Check sheet for the drawn part. Datum: minimum x, y, z corner. Units: mm. A direction names the side the tool comes from. Round coordinates to 2 decimals unless told otherwise and drop trailing zeros. Order: outer loops, then holes, each group sorted by start corner. A loop starts at its lowest first (then second) coordinate and runs counter-clockwise, first axis right, second up. Notation, with made-up numbers: (-21.75, 71.25) -> (22.25, 71.25) arc R31 ccw to (22.25, 98.25) -> close; hole circle Ø1 at (0.5, -25.75). An arc over 180 degrees is marked (long way). Answer in a Markdown table with one row per item.
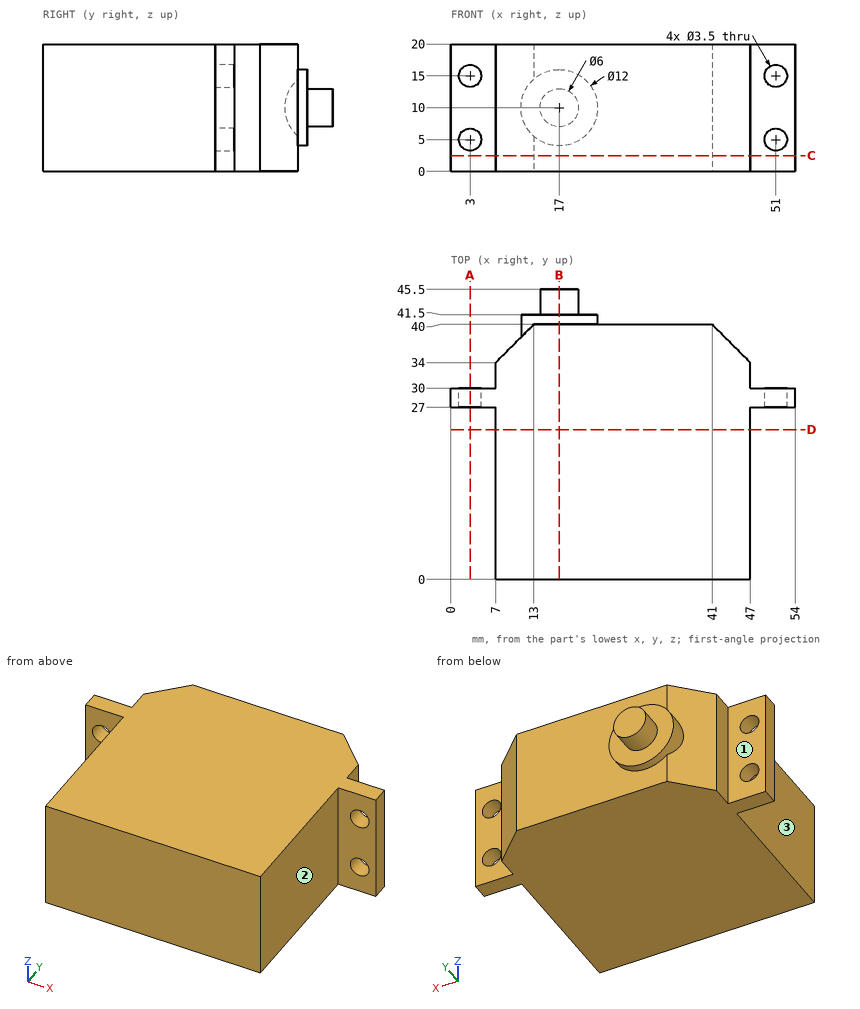
(1) Tool access check on the marked faces 1, 2 and 3. Record the directions out of +Z, -Z, +X, -X, +Y, -Y that give a thin tool (end or side, any length) a straight path to the whole face; none if there is none.
Solutions:
| item | result |
|---|---|
| face 1 | +Z, -Z, -X, +Y |
| face 2 | +Z, -Z, +X, -Y |
| face 3 | +Z, -Z, -X, -Y |
(2) Scan lines: probe 1 along X at (y, z) = (28.2, 15); probe 2 along Y at (x, z) = (13.5, 16.75); probe 3 along Y at (x, z) = (16, 15.75). Record each from-to range of solid material in increasing order. Write a range as from..to.
Solutions:
| item | result |
|---|---|
| probe 1 | 0..1.25, 4.75..49.25, 52.75..54 |
| probe 2 | 0..40 |
| probe 3 | 0..41.5 |
(3) Section check A-A on x = 3. Record the boundary of the cut face in (y, z).
Solutions:
| item | result |
|---|---|
| outline | (27, 0) -> (30, 0) -> (30, 3.25) -> (27, 3.25) -> close; (27, 6.75) -> (30, 6.75) -> (30, 13.25) -> (27, 13.25) -> close; (27, 16.75) -> (30, 16.75) -> (30, 20) -> (27, 20) -> close |
(4) Section check D-D on y = 23.5. Record the boundary of the cut face in (x, z), plus the area to 3 significant figures.
Solutions:
| item | result |
|---|---|
| outline | (7, 0) -> (47, 0) -> (47, 20) -> (7, 20) -> close |
| area | 800 mm^2 |
(5) Section check B-B on x = 17. Record the boundary of the cut face in (y, z), plus the area to 3 significant figures.
Solutions:
| item | result |
|---|---|
| outline | (0, 0) -> (40, 0) -> (40, 4) -> (41.5, 4) -> (41.5, 7) -> (45.5, 7) -> (45.5, 13) -> (41.5, 13) -> (41.5, 16) -> (40, 16) -> (40, 20) -> (0, 20) -> close |
| area | 842 mm^2 |
(6) Depth check by flat-ended pin: pin 1 Ø3 at (y, z) = (32, 6.5) entering from -X; pin 2 Ø5.5 at (x, z) = (50.5, 15) entering from +Y; pin 3 Ø7.5 at (x, z) = (3, 10) entering from -Y; pin 4 Ø3 at (x, z) = (51, 15) entering from -Y. Enter the tip coordinate at first touch or a pass-through.
Solutions:
| item | result |
|---|---|
| pin 1 | x = 7 |
| pin 2 | y = 30 |
| pin 3 | y = 27 |
| pin 4 | through |
(7) Section check C-C on z = 2.5. Record the boundary of the cut face in (x, y), plus the area to 3 significant figures.
Solutions:
| item | result |
|---|---|
| outline | (0, 27) -> (7, 27) -> (7, 0) -> (47, 0) -> (47, 27) -> (54, 27) -> (54, 30) -> (47, 30) -> (47, 34) -> (41, 40) -> (13, 40) -> (7, 34) -> (7, 30) -> (0, 30) -> close |
| area | 1,610 mm^2 |
